```python
from build123d import *

# Parameters (mm, degrees)
BOSS_EXTRUDE1_DEPTH      = 2.3876
BOSS_EXTRUDE1_DEPTH_BACK = 2.3876
SKETCH4_R                = 3.2639
CUT_EXTRUDE1_DEPTH       = 1
CUT_EXTRUDE1_DEPTH_BACK  = 5.7752
SKETCH5_R                = 3.2639
CUT_EXTRUDE2_DEPTH       = 5.7752


with BuildPart() as part:
    # Sketch3 → Boss-Extrude1 (new body, two sides)
    with BuildSketch(Plane.XY) as boss_extrude1_sk:
        Polygon((-12.7, 63.5), (12.7, 63.5), (38.1, 12.7), (38.1, -12.7), (12.7, -63.5), (-12.7, -63.5), (-38.1, -12.7), (-38.1, 12.7), align=None)
    extrude(amount=BOSS_EXTRUDE1_DEPTH)
    extrude(boss_extrude1_sk.sketch, amount=-BOSS_EXTRUDE1_DEPTH_BACK)

    # Sketch4 → Cut-Extrude1 (cut, two sides)
    with BuildSketch(Plane.XY.offset(2.3876)) as cut_extrude1_sk:
        with Locations((0, 50.8)):
            Circle(SKETCH4_R)
        with Locations((0, 25.4)):
            Circle(SKETCH4_R)
        Circle(SKETCH4_R)
        with Locations((0, -25.4)):
            Circle(SKETCH4_R)
        with Locations((0, -50.8)):
            Circle(SKETCH4_R)
    extrude(amount=CUT_EXTRUDE1_DEPTH, mode=Mode.SUBTRACT)
    extrude(cut_extrude1_sk.sketch, amount=-CUT_EXTRUDE1_DEPTH_BACK, mode=Mode.SUBTRACT)

    # Sketch5 → Cut-Extrude2 (cut, through all)
    with BuildSketch(Plane.XY.offset(2.3876)):
        with Locations((25.4, 0)):
            Circle(SKETCH5_R)
        with Locations((-25.4, 0)):
            Circle(SKETCH5_R)
    extrude(amount=-CUT_EXTRUDE2_DEPTH, mode=Mode.SUBTRACT)


solid = part.part
```
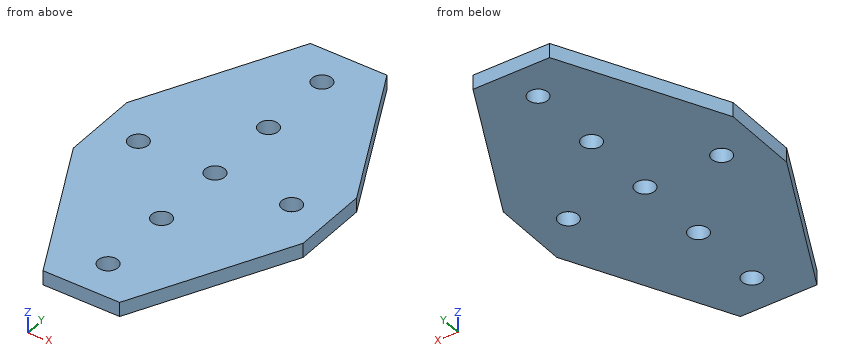
The model under review builds one solid part; all positions refer to its coordinate system, in mm. Give positions to 0.01 mm unless a question says otherwise; leave off trailing zeros. Write each loop counter-clockwise with the first axis right and the second up, starting at its lowest first coordinate (ties: lowest second). Pieces come first, ordered by that corner, then holes.
(1) Consider section D-D, the plane x = -25.4. Give the boundary of the cut face in (y, z), and give its area (3 significant figures).
(2) To check wall thickness, follow L1, parallel to Y at x = 0, z = -0.6; L2, parallel to Y at x = -25.4, z = 1.4; L3, parallel to Y at x = -2.5, z = 0.9. State the ranges of each line that lie inside material, in increasing order.
(3) Consider section A-A, the plane y = -50.8. Give the boundary of the cut face in (x, z).
(4) For P1, Ø6, axis at x = 0, y = -50.8, coming from the -Z side; P2, Ø1, axis at x = 14, z = 1, coming from the +Y side, all flat-tipped, find the tip position at first contact; note any pin that passes through.
(5) Consider section C-C, the plane y = 0. Give the boundary of the cut face in (x, z), and give its area (3 significant figures).
(6) Consider section B-B, the plane x = 0. Give the boundary of the cut face in (y, z), and give its area (3 significant figures).
Returned:
1. outline: (-38.1, -2.39) - (-3.26, -2.39) - (-3.26, 2.39) - (-38.1, 2.39) - close; (3.26, -2.39) - (38.1, -2.39) - (38.1, 2.39) - (3.26, 2.39) - close
1. area: 333 mm2
2. L1: y = -63.5 to -54.06, -47.54 to -28.66, -22.14 to -3.26, 3.26 to 22.14, 28.66 to 47.54, 54.06 to 63.5
2. L2: y = -38.1 to -3.26, 3.26 to 38.1
2. L3: y = -63.5 to -52.9, -48.7 to -27.5, -23.3 to -2.1, 2.1 to 23.3, 27.5 to 48.7, 52.9 to 63.5
3. outline: (-19.05, -2.39) - (-3.26, -2.39) - (-3.26, 2.39) - (-19.05, 2.39) - close; (3.26, -2.39) - (19.05, -2.39) - (19.05, 2.39) - (3.26, 2.39) - close
4. P1: passes through
4. P2: stops at y = 61.9
5. outline: (-38.1, -2.39) - (-28.66, -2.39) - (-28.66, 2.39) - (-38.1, 2.39) - close; (-22.14, -2.39) - (-3.26, -2.39) - (-3.26, 2.39) - (-22.14, 2.39) - close; (3.26, -2.39) - (22.14, -2.39) - (22.14, 2.39) - (3.26, 2.39) - close; (28.66, -2.39) - (38.1, -2.39) - (38.1, 2.39) - (28.66, 2.39) - close
5. area: 270 mm2
6. outline: (-63.5, -2.39) - (-54.06, -2.39) - (-54.06, 2.39) - (-63.5, 2.39) - close; (-47.54, -2.39) - (-28.66, -2.39) - (-28.66, 2.39) - (-47.54, 2.39) - close; (-22.14, -2.39) - (-3.26, -2.39) - (-3.26, 2.39) - (-22.14, 2.39) - close; (3.26, -2.39) - (22.14, -2.39) - (22.14, 2.39) - (3.26, 2.39) - close; (28.66, -2.39) - (47.54, -2.39) - (47.54, 2.39) - (28.66, 2.39) - close; (54.06, -2.39) - (63.5, -2.39) - (63.5, 2.39) - (54.06, 2.39) - close
6. area: 451 mm2
